Can you work these out from the model? Positions are in its coordinate system, mm. A direction names the side the tool comes from. Round coordinates to 2 decimals unless told otherwise and drop trailing zeros. Write each loop counter-clockwise with the first axis right and the second up, starting at its lowest first coordinate (ties: lowest second). Pieces come first, ordered by that corner, then holes.
Q1. I'm going to push flat-ended pins straight in: pin 1 Ø8 at (x, z) = (22, -7) entering from -Y; pin 2 Ø8 at (y, z) = (3.5, 19) entering from +X; pin 3 Ø16.5 at (y, z) = (-32, -2.5) entering from -X. Where does each tip first touch, or does it pass through?
Q2. For faces 5 (the flat face through (-6, -40.7, -0.3)), 6 (the flat face through (25, -32, 0)), 7 (the flat face through (-15, -40.7, -0.3)), which set-ups out of +Z, -Z, +X, -X, +Y, -Y let a thin tool reach every point of the face, with its end or its side?
Q3. If we section it at C-C (z = 12.5): Please give me the cut outline in (x, y).
Q4. If we section it at B-B (y = -47): Please give me the cut outline in (x, z), plus the area to 3 significant figures.
Q5. If we section it at D-D (y = -29.5): Please give me the cut outline in (x, z).
Q6. If we section it at A-A (x = 8.5): Please give me the cut outline in (y, z), plus the area to 3 significant figures.
Q7. Please list where these lines run through material, in increasing order: line 1 along X through (y, z) = (-46.5, -12.5); line 2 along Y through (x, z) = (-41, -16); line 3 along Z through (x, y) = (9.25, -47).
Q8. We'd pull the mould along Z, two halves only. Please class faces 1 (the cylindrical face through (-10, -53, 0)), 2 (the flat face through (61, -25, 0)), 3 (the cylindrical face through (0.35, -36.524, 24.942)), 4 (the cylindrical face through (-94.906, -0.35, 0.55)): +Z half, -Z half, draft (parallel to the pull), parting line (faces both ways), or undercut.
from build123d import *

# Parameters (mm, degrees)
F1_DEPTH  = 25
F2_W      = 50
F2_H      = 50
F3_DEPTH  = 30
F6_W      = 6
F6_H      = 15
F5_W      = 6
F5_H      = 15
F4_W      = 10
F4_H      = 15
F7_DEPTH  = 50.001
F8_F1_R   = 20
F8_F2_R   = 20
F9_R      = 6
F10_DEPTH = 134.901


with BuildPart() as f1:
    # F0 (on Front) → F1 (new body, symmetric)
    with BuildSketch(Plane.XZ):
        with BuildLine():
            Line((-119.9, -25), (119.9, -25))
            ThreePointArc((119.9, -25), (94.9, 0), (119.9, 25))
            Line((119.9, 25), (-119.9, 25))
            ThreePointArc((-119.9, 25), (-94.9, 0), (-119.9, -25))
        make_face()
    extrude(amount=F1_DEPTH, both=True)

    # F2 (on face) → F3 (join)
    with BuildSketch(Plane.XZ.offset(25)):
        Rectangle(F2_W, F2_H)
    extrude(amount=F3_DEPTH)

    # F6 (on face) + F5 (on face) + F4 (on face) → F7 (cut, through all)
    with BuildSketch(Plane(origin=(0, 0, -25), x_dir=(1, 0, 0), z_dir=(0, 0, -1))):
        with Locations((-3, 47.5)):
            Rectangle(F6_W, F6_H)
    with BuildSketch(Plane(origin=(0, 0, -25), x_dir=(1, 0, 0), z_dir=(0, 0, -1))):
        with Locations((3, 47.5)):
            Rectangle(F5_W, F5_H)
    with BuildSketch(Plane(origin=(0, 0, -25), x_dir=(1, 0, 0), z_dir=(0, 0, -1))):
        with Locations((20, 47.5)):
            Rectangle(F4_W, F4_H)
        with Locations((-20, 47.5)):
            Rectangle(F4_W, F4_H)
    extrude(amount=-F7_DEPTH, mode=Mode.SUBTRACT)

    # F8: fillet of radius 20 on 4 edges, made by hand

    # F8_f1
    f8_f1_edges = [f1.edges().sort_by_distance(p)[0] for p in [
        (10.5, -55, 25),
    ]]
    fillet(f8_f1_edges, radius=F8_F1_R)

    # F8_f2
    f8_f2_edges = [f1.edges().sort_by_distance(p)[0] for p in [
        (10.5, -55, -25),
    ]]
    fillet(f8_f2_edges, radius=F8_F2_R)

    # F9 (on face) → F10 (cut, through all)
    with BuildSketch(Plane.YZ.offset(15)):
        with Locations((-47, 0)):
            Circle(F9_R)
    extrude(amount=-F10_DEPTH, mode=Mode.SUBTRACT)


solid = f1.part
A:
1. pin 1: stops at y = -40
1. pin 2: stops at x = 110.1
1. pin 3: stops at x = -95.86
2. face 5: +Z, -Z, -Y
2. face 6: +Z, -Z, +X, -Y
2. face 7: +Z, -Z, -X, -Y
3. outline: (-98.25, -25) - (-25, -25) - (-25, -40) - (-15, -40) - (-15, -53.54) - (-6, -53.54) - (-6, -40) - (6, -40) - (6, -53.54) - (15, -53.54) - (15, -40) - (25, -40) - (25, -25) - (98.25, -25) - (98.25, 25) - (-98.25, 25) - close
4. outline: (-15, -21) - (-6, -21) - (-6, -6) - (-15, -6) - close; (-15, 6) - (-6, 6) - (-6, 21) - (-15, 21) - close; (6, -21) - (15, -21) - (15, -6) - (6, -6) - close; (6, 6) - (15, 6) - (15, 21) - (6, 21) - close
4. area: 540 mm2
5. outline: (-25, -25) - (25, -25) - (25, 25) - (-25, 25) - close
6. outline: (-55, -5) arc R20 ccw to (-35, -25) - (25, -25) - (25, 25) - (-35, 25) arc R20 ccw to (-55, 5) - close; hole circle Ø12 at (-47, 0)
6. area: 3,720 mm2
7. line 1: x = -15 to -6, 6 to 15
7. line 2: y = -25 to 25
7. line 3: z = -21 to -6, 6 to 21
8. face 1: undercut
8. face 2: draft
8. face 3: +Z half
8. face 4: undercut
